from build123d import *

# Parameters (mm, degrees)
CYLINDER028_R               = 1
CYLINDER028_DEPTH           = 15
CYLINDER028_ROLL_ANGLE      = 90.000024
CYLINDER028_PITCH_ANGLE     = -1e-05
CYLINDER028_PLACEMENT_ANGLE = 45.000049
CYLINDER027_R               = 5.5
CYLINDER027_DEPTH           = 3
CYLINDER020_R               = 2.5
CYLINDER020_DEPTH           = 60
CYLINDER019_R               = 5.5
CYLINDER019_DEPTH           = 10
BOX001_W                    = 65
BOX001_H                    = 65
BOX001_DEPTH                = 5


with BuildPart() as kegel025:
    # Cone025 → Cone025 (revolve)
    with BuildSketch(Plane(origin=(-15.75, -26.25, 78), x_dir=(1, 0, 0), z_dir=(0, -1, 0))):
        Polygon((0, 0), (3.25, 0), (3.5, 5), (0, 5), align=None)
    revolve(axis=Axis((-15.75, -26.25, 78), (0, 0, 1)))


with BuildPart() as kegel026:
    # Cone026 → Cone026 (revolve)
    with BuildSketch(Plane(origin=(-26.25, -26.25, 78), x_dir=(1, 0, 0), z_dir=(0, -1, 0))):
        Polygon((0, 0), (3.25, 0), (3.5, 5), (0, 5), align=None)
    revolve(axis=Axis((-26.25, -26.25, 78), (0, 0, 1)))


with BuildPart() as kegel027:
    # Cone027 → Cone027 (revolve)
    with BuildSketch(Plane(origin=(-26.25, -15.75, 78), x_dir=(1, 0, 0), z_dir=(0, -1, 0))):
        Polygon((0, 0), (3.25, 0), (3.5, 5), (0, 5), align=None)
    revolve(axis=Axis((-26.25, -15.75, 78), (0, 0, 1)))


with BuildPart() as kegel028:
    # Cone028 → Cone028 (revolve)
    with BuildSketch(Plane(origin=(-26.25, -5.25, 78), x_dir=(1, 0, 0), z_dir=(0, -1, 0))):
        Polygon((0, 0), (3.25, 0), (3.5, 5), (0, 5), align=None)
    revolve(axis=Axis((-26.25, -5.25, 78), (0, 0, 1)))


with BuildPart() as kegel029:
    # Cone029 → Cone029 (revolve)
    with BuildSketch(Plane(origin=(-26.25, 5.25, 78), x_dir=(1, 0, 0), z_dir=(0, -1, 0))):
        Polygon((0, 0), (3.25, 0), (3.5, 5), (0, 5), align=None)
    revolve(axis=Axis((-26.25, 5.25, 78), (0, 0, 1)))


with BuildPart() as kegel030:
    # Cone030 → Cone030 (revolve)
    with BuildSketch(Plane(origin=(-26.25, 15.75, 78), x_dir=(1, 0, 0), z_dir=(0, -1, 0))):
        Polygon((0, 0), (3.25, 0), (3.5, 5), (0, 5), align=None)
    revolve(axis=Axis((-26.25, 15.75, 78), (0, 0, 1)))


with BuildPart() as kegel031:
    # Cone031 → Cone031 (revolve)
    with BuildSketch(Plane(origin=(-26.25, 26.25, 78), x_dir=(1, 0, 0), z_dir=(0, -1, 0))):
        Polygon((0, 0), (3.25, 0), (3.5, 5), (0, 5), align=None)
    revolve(axis=Axis((-26.25, 26.25, 78), (0, 0, 1)))


with BuildPart() as kegel024:
    # Cone024 → Cone024 (revolve)
    with BuildSketch(Plane(origin=(-5.25, -26.25, 78), x_dir=(1, 0, 0), z_dir=(0, -1, 0))):
        Polygon((0, 0), (3.25, 0), (3.5, 5), (0, 5), align=None)
    revolve(axis=Axis((-5.25, -26.25, 78), (0, 0, 1)))


with BuildPart() as zylinder026:
    # Cylinder028 → Cylinder028 (new body)
    with BuildSketch(Plane.XY):
        Circle(CYLINDER028_R)
    extrude(amount=CYLINDER028_DEPTH)


with BuildPart() as zylinder026_1:
    # Cylinder028 roll: moved
    add(zylinder026.part.rotate(Axis((0, 0, 0), (1, 0, 0)), CYLINDER028_ROLL_ANGLE))


with BuildPart() as zylinder026_2:
    # Cylinder028 pitch: moved
    add(zylinder026_1.part.rotate(Axis((0, 0, 0), (0, 1, 0)), CYLINDER028_PITCH_ANGLE))


with BuildPart() as zylinder026_3:
    # Cylinder028 placement: moved
    add(zylinder026_2.part.moved(Location((-6, 6, 90))).rotate(Axis((-6, 6, 90), (0, 0, 1)), CYLINDER028_PLACEMENT_ANGLE))


with BuildPart() as zylinder025:
    # Cylinder027 → Cylinder027 (new body)
    with BuildSketch(Plane.XY.offset(93)):
        Circle(CYLINDER027_R)
    extrude(amount=CYLINDER027_DEPTH)


with BuildPart() as spindel001:
    # Cylinder020 → Cylinder020 (new body)
    with BuildSketch(Plane.XY.offset(33)):
        Circle(CYLINDER020_R)
    extrude(amount=CYLINDER020_DEPTH)


with BuildPart() as zylinder018:
    # Cylinder019 → Cylinder019 (new body)
    with BuildSketch(Plane.XY.offset(83)):
        Circle(CYLINDER019_R)
    extrude(amount=CYLINDER019_DEPTH)


with BuildPart() as kegel001:
    # Cone001 → Cone001 (revolve)
    with BuildSketch(Plane(origin=(26.25, 15.75, 78), x_dir=(1, 0, 0), z_dir=(0, -1, 0))):
        Polygon((0, 0), (3.25, 0), (3.5, 5), (0, 5), align=None)
    revolve(axis=Axis((26.25, 15.75, 78), (0, 0, 1)))


with BuildPart() as kegel002:
    # Cone002 → Cone002 (revolve)
    with BuildSketch(Plane(origin=(26.25, 5.25, 78), x_dir=(1, 0, 0), z_dir=(0, -1, 0))):
        Polygon((0, 0), (3.25, 0), (3.5, 5), (0, 5), align=None)
    revolve(axis=Axis((26.25, 5.25, 78), (0, 0, 1)))


with BuildPart() as kegel003:
    # Cone003 → Cone003 (revolve)
    with BuildSketch(Plane(origin=(26.25, -5.25, 78), x_dir=(1, 0, 0), z_dir=(0, -1, 0))):
        Polygon((0, 0), (3.25, 0), (3.5, 5), (0, 5), align=None)
    revolve(axis=Axis((26.25, -5.25, 78), (0, 0, 1)))


with BuildPart() as kegel004:
    # Cone004 → Cone004 (revolve)
    with BuildSketch(Plane(origin=(15.75, -15.75, 78), x_dir=(1, 0, 0), z_dir=(0, -1, 0))):
        Polygon((0, 0), (3.25, 0), (3.5, 5), (0, 5), align=None)
    revolve(axis=Axis((15.75, -15.75, 78), (0, 0, 1)))


with BuildPart() as kegel005:
    # Cone005 → Cone005 (revolve)
    with BuildSketch(Plane(origin=(26.25, -15.75, 78), x_dir=(1, 0, 0), z_dir=(0, -1, 0))):
        Polygon((0, 0), (3.25, 0), (3.5, 5), (0, 5), align=None)
    revolve(axis=Axis((26.25, -15.75, 78), (0, 0, 1)))


with BuildPart() as kegel006:
    # Cone006 → Cone006 (revolve)
    with BuildSketch(Plane(origin=(15.75, -5.25, 78), x_dir=(1, 0, 0), z_dir=(0, -1, 0))):
        Polygon((0, 0), (3.25, 0), (3.5, 5), (0, 5), align=None)
    revolve(axis=Axis((15.75, -5.25, 78), (0, 0, 1)))


with BuildPart() as kegel007:
    # Cone007 → Cone007 (revolve)
    with BuildSketch(Plane(origin=(15.75, 5.25, 78), x_dir=(1, 0, 0), z_dir=(0, -1, 0))):
        Polygon((0, 0), (3.25, 0), (3.5, 5), (0, 5), align=None)
    revolve(axis=Axis((15.75, 5.25, 78), (0, 0, 1)))


with BuildPart() as kegel008:
    # Cone008 → Cone008 (revolve)
    with BuildSketch(Plane(origin=(15.75, 15.75, 78), x_dir=(1, 0, 0), z_dir=(0, -1, 0))):
        Polygon((0, 0), (3.25, 0), (3.5, 5), (0, 5), align=None)
    revolve(axis=Axis((15.75, 15.75, 78), (0, 0, 1)))


with BuildPart() as kegel009:
    # Cone009 → Cone009 (revolve)
    with BuildSketch(Plane(origin=(15.75, 26.25, 78), x_dir=(1, 0, 0), z_dir=(0, -1, 0))):
        Polygon((0, 0), (3.25, 0), (3.5, 5), (0, 5), align=None)
    revolve(axis=Axis((15.75, 26.25, 78), (0, 0, 1)))


with BuildPart() as kegel010:
    # Cone010 → Cone010 (revolve)
    with BuildSketch(Plane(origin=(5.25, -15.75, 78), x_dir=(1, 0, 0), z_dir=(0, -1, 0))):
        Polygon((0, 0), (3.25, 0), (3.5, 5), (0, 5), align=None)
    revolve(axis=Axis((5.25, -15.75, 78), (0, 0, 1)))


with BuildPart() as kegel011:
    # Cone011 → Cone011 (revolve)
    with BuildSketch(Plane(origin=(-5.25, -15.75, 78), x_dir=(1, 0, 0), z_dir=(0, -1, 0))):
        Polygon((0, 0), (3.25, 0), (3.5, 5), (0, 5), align=None)
    revolve(axis=Axis((-5.25, -15.75, 78), (0, 0, 1)))


with BuildPart() as kegel012:
    # Cone012 → Cone012 (revolve)
    with BuildSketch(Plane(origin=(-15.75, -15.75, 78), x_dir=(1, 0, 0), z_dir=(0, -1, 0))):
        Polygon((0, 0), (3.25, 0), (3.5, 5), (0, 5), align=None)
    revolve(axis=Axis((-15.75, -15.75, 78), (0, 0, 1)))


with BuildPart() as kegel013:
    # Cone013 → Cone013 (revolve)
    with BuildSketch(Plane(origin=(-15.75, -5.25, 78), x_dir=(1, 0, 0), z_dir=(0, -1, 0))):
        Polygon((0, 0), (3.25, 0), (3.5, 5), (0, 5), align=None)
    revolve(axis=Axis((-15.75, -5.25, 78), (0, 0, 1)))


with BuildPart() as kegel014:
    # Cone014 → Cone014 (revolve)
    with BuildSketch(Plane(origin=(-15.75, 5.25, 78), x_dir=(1, 0, 0), z_dir=(0, -1, 0))):
        Polygon((0, 0), (3.25, 0), (3.5, 5), (0, 5), align=None)
    revolve(axis=Axis((-15.75, 5.25, 78), (0, 0, 1)))


with BuildPart() as kegel015:
    # Cone015 → Cone015 (revolve)
    with BuildSketch(Plane(origin=(-15.75, 15.75, 78), x_dir=(1, 0, 0), z_dir=(0, -1, 0))):
        Polygon((0, 0), (3.25, 0), (3.5, 5), (0, 5), align=None)
    revolve(axis=Axis((-15.75, 15.75, 78), (0, 0, 1)))


with BuildPart() as kegel016:
    # Cone016 → Cone016 (revolve)
    with BuildSketch(Plane(origin=(-15.75, 26.25, 78), x_dir=(1, 0, 0), z_dir=(0, -1, 0))):
        Polygon((0, 0), (3.25, 0), (3.5, 5), (0, 5), align=None)
    revolve(axis=Axis((-15.75, 26.25, 78), (0, 0, 1)))


with BuildPart() as kegel017:
    # Cone017 → Cone017 (revolve)
    with BuildSketch(Plane(origin=(-5.25, 26.25, 78), x_dir=(1, 0, 0), z_dir=(0, -1, 0))):
        Polygon((0, 0), (3.25, 0), (3.5, 5), (0, 5), align=None)
    revolve(axis=Axis((-5.25, 26.25, 78), (0, 0, 1)))


with BuildPart() as kegel018:
    # Cone018 → Cone018 (revolve)
    with BuildSketch(Plane(origin=(5.25, 26.25, 78), x_dir=(1, 0, 0), z_dir=(0, -1, 0))):
        Polygon((0, 0), (3.25, 0), (3.5, 5), (0, 5), align=None)
    revolve(axis=Axis((5.25, 26.25, 78), (0, 0, 1)))


with BuildPart() as kegel019:
    # Cone019 → Cone019 (revolve)
    with BuildSketch(Plane(origin=(-5.25, 15.75, 78), x_dir=(1, 0, 0), z_dir=(0, -1, 0))):
        Polygon((0, 0), (3.25, 0), (3.5, 5), (0, 5), align=None)
    revolve(axis=Axis((-5.25, 15.75, 78), (0, 0, 1)))


with BuildPart() as kegel020:
    # Cone020 → Cone020 (revolve)
    with BuildSketch(Plane(origin=(5.25, 15.75, 78), x_dir=(1, 0, 0), z_dir=(0, -1, 0))):
        Polygon((0, 0), (3.25, 0), (3.5, 5), (0, 5), align=None)
    revolve(axis=Axis((5.25, 15.75, 78), (0, 0, 1)))


with BuildPart() as kegel021:
    # Cone021 → Cone021 (revolve)
    with BuildSketch(Plane(origin=(5.25, -26.25, 78), x_dir=(1, 0, 0), z_dir=(0, -1, 0))):
        Polygon((0, 0), (3.25, 0), (3.5, 5), (0, 5), align=None)
    revolve(axis=Axis((5.25, -26.25, 78), (0, 0, 1)))


with BuildPart() as kegel022:
    # Cone022 → Cone022 (revolve)
    with BuildSketch(Plane(origin=(15.75, -26.25, 78), x_dir=(1, 0, 0), z_dir=(0, -1, 0))):
        Polygon((0, 0), (3.25, 0), (3.5, 5), (0, 5), align=None)
    revolve(axis=Axis((15.75, -26.25, 78), (0, 0, 1)))


with BuildPart() as kegel023:
    # Cone023 → Cone023 (revolve)
    with BuildSketch(Plane(origin=(26.25, -26.25, 78), x_dir=(1, 0, 0), z_dir=(0, -1, 0))):
        Polygon((0, 0), (3.25, 0), (3.5, 5), (0, 5), align=None)
    revolve(axis=Axis((26.25, -26.25, 78), (0, 0, 1)))


with BuildPart() as kegel:
    # Cone → Cone (revolve)
    with BuildSketch(Plane(origin=(26.25, 26.25, 78), x_dir=(1, 0, 0), z_dir=(0, -1, 0))):
        Polygon((0, 0), (3.25, 0), (3.5, 5), (0, 5), align=None)
    revolve(axis=Axis((26.25, 26.25, 78), (0, 0, 1)))


with BuildPart() as top001:
    # Box001 → Box001 (new body)
    with BuildSketch(Plane(origin=(-32.5, -32.5, 78), x_dir=(1, 0, 0), z_dir=(0, 0, 1))):
        with Locations((32.5, 32.5)):
            Rectangle(BOX001_W, BOX001_H)
    extrude(amount=BOX001_DEPTH)

    # Cut008: cut Kegel
    add(kegel.part, mode=Mode.SUBTRACT)

    # Cut009: cut Kegel023
    add(kegel023.part, mode=Mode.SUBTRACT)

    # Cut010: cut Kegel022
    add(kegel022.part, mode=Mode.SUBTRACT)

    # Cut011: cut Kegel021
    add(kegel021.part, mode=Mode.SUBTRACT)

    # Cut012: cut Kegel020
    add(kegel020.part, mode=Mode.SUBTRACT)

    # Cut013: cut Kegel019
    add(kegel019.part, mode=Mode.SUBTRACT)

    # Cut014: cut Kegel018
    add(kegel018.part, mode=Mode.SUBTRACT)

    # Cut015: cut Kegel017
    add(kegel017.part, mode=Mode.SUBTRACT)

    # Cut016: cut Kegel016
    add(kegel016.part, mode=Mode.SUBTRACT)

    # Cut017: cut Kegel015
    add(kegel015.part, mode=Mode.SUBTRACT)

    # Cut018: cut Kegel014
    add(kegel014.part, mode=Mode.SUBTRACT)

    # Cut019: cut Kegel013
    add(kegel013.part, mode=Mode.SUBTRACT)

    # Cut020: cut Kegel012
    add(kegel012.part, mode=Mode.SUBTRACT)

    # Cut021: cut Kegel011
    add(kegel011.part, mode=Mode.SUBTRACT)

    # Cut022: cut Kegel010
    add(kegel010.part, mode=Mode.SUBTRACT)

    # Cut023: cut Kegel009
    add(kegel009.part, mode=Mode.SUBTRACT)

    # Cut024: cut Kegel008
    add(kegel008.part, mode=Mode.SUBTRACT)

    # Cut025: cut Kegel007
    add(kegel007.part, mode=Mode.SUBTRACT)

    # Cut026: cut Kegel006
    add(kegel006.part, mode=Mode.SUBTRACT)

    # Cut027: cut Kegel005
    add(kegel005.part, mode=Mode.SUBTRACT)

    # Cut028: cut Kegel004
    add(kegel004.part, mode=Mode.SUBTRACT)

    # Cut029: cut Kegel003
    add(kegel003.part, mode=Mode.SUBTRACT)

    # Cut030: cut Kegel002
    add(kegel002.part, mode=Mode.SUBTRACT)

    # Cut031: cut Kegel001
    add(kegel001.part, mode=Mode.SUBTRACT)

    # Fusion: union Zylinder018
    add(zylinder018.part)

    # Cut032: cut Spindel001
    add(spindel001.part, mode=Mode.SUBTRACT)

    # Fusion002: union Zylinder025
    add(zylinder025.part)

    # Cut042: cut Zylinder026
    add(zylinder026_3.part, mode=Mode.SUBTRACT)

    # Cut048: cut Kegel024
    add(kegel024.part, mode=Mode.SUBTRACT)

    # Cut049: cut Kegel031
    add(kegel031.part, mode=Mode.SUBTRACT)

    # Cut050: cut Kegel030
    add(kegel030.part, mode=Mode.SUBTRACT)

    # Cut051: cut Kegel029
    add(kegel029.part, mode=Mode.SUBTRACT)

    # Cut052: cut Kegel028
    add(kegel028.part, mode=Mode.SUBTRACT)

    # Cut053: cut Kegel027
    add(kegel027.part, mode=Mode.SUBTRACT)

    # Cut054: cut Kegel026
    add(kegel026.part, mode=Mode.SUBTRACT)

    # Cut055: cut Kegel025
    add(kegel025.part, mode=Mode.SUBTRACT)


solid = top001.part
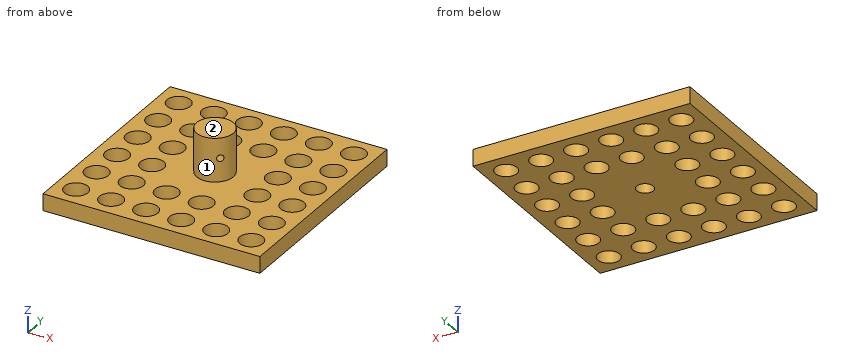
Source: CAD feature listing. Evaluate the final solid. Frame: model axes, mm. Face numbers are marked on the shaded views. A direction names the side the tool comes from. Give positions to 0.01 mm unless a question says otherwise; leave off trailing zeros. Loops run counter-clockwise (first coordinate to the right, second up) from the corner with the lowest first, then second, coordinate; pieces in that order, holes last. Notation, with made-up numbers: (-33.75, 39.5) -> (19.25, 39.5) arc R25 ccw to (19.25, 69.5) -> close; hole circle Ø8 at (-26, 7.5). An arc over 180 degrees is marked (long way). Use a Markdown table: item, result. Add a question column.
1) Line query: line 1 along Y through (x, z) = (0, 90); line 2 along Z through (x, y) = (9.5, 12.5); line 3 along X through (y, z) = (-4, 89.25). Output: solid intervals per line, ascending. Write a range as [from, to].
2) Section query D-D, the plane z = 85. Return the cut outline in (x, y).
3) First-contact query: pin 1 (6 mm diameter, centred on x = -25.5, y = -4, fed in from +Z); pin 2 (1.5 mm diameter, centred on x = 0, y = -0.5, fed in from -Z); pin 3 (1.5 mm diameter, centred on y = -3, z = 90.5, fed in from -X). Flat tips, straight axial feed; report the tip coordinate or a pass-through.
4) Reachability of the marked faces 1 and 2 from +Z, -Z, +X, -X, +Y, -Y: full face, straight path, thin tool, end or side. Return the list, or none.
5) Section query C-C, the plane x = 0. Return the cut outline in (y, z).
6) Section query A-A, the plane x = -26.25. Return the cut outline in (y, z), then the cut area to 4 significant figures.
Numbers:
| question | item | result |
|---|---|---|
| 1 | line 1 | y = [-5.5, -2.5], [2.5, 5.5] |
| 1 | line 2 | z = [78, 83] |
| 1 | line 3 | x = [-3.77, 3.06] |
| 2 | outline | circle Ø11 at (0, 0); hole circle Ø5 at (0, 0) |
| 3 | pin 1 | stops at z = 83 |
| 3 | pin 2 | stops at z = 93 |
| 3 | pin 3 | stops at x = -5.02 |
| 4 | face 1 | +Z |
| 4 | face 2 | +Z, +X, -X, +Y, -Y |
| 5 | outline | (-32.5, 78) -> (-2.5, 78) -> (-2.5, 93) -> (2.5, 93) -> (2.5, 78) -> (32.5, 78) -> (32.5, 83) -> (5.5, 83) -> (5.5, 96) -> (-5.5, 96) -> (-5.5, 83) -> (-32.5, 83) -> close |
| 6 | outline | (-32.5, 78) -> (-29.5, 78) -> (-29.75, 83) -> (-32.5, 83) -> close; (-23, 78) -> (-19, 78) -> (-19.25, 83) -> (-22.75, 83) -> close; (-12.5, 78) -> (-8.5, 78) -> (-8.75, 83) -> (-12.25, 83) -> close; (-2, 78) -> (2, 78) -> (1.75, 83) -> (-1.75, 83) -> close; (8.5, 78) -> (12.5, 78) -> (12.25, 83) -> (8.75, 83) -> close; (19, 78) -> (23, 78) -> (22.75, 83) -> (19.25, 83) -> close; (29.5, 78) -> (32.5, 78) -> (32.5, 83) -> (29.75, 83) -> close |
| 6 | area | 122.5 mm2 |
